Geometry check sheet. Reference: the model listing, model coordinates, mm. Face numbers are marked on the shaded views. Give positions to 0.01 mm unless a question says otherwise; leave off trailing zeros. Write each loop counter-clockwise with the first axis right and the second up, starting at its lowest first coordinate (ties: lowest second). Pieces come first, ordered by that corner, then holes. Notation, with made-up numbers: M -19,33.5 L 0,33.5 A16 cw 0,46.5 Z; hole C 9.5,87.25 d11. An arc over 180 degrees is marked long. Write each question's results on one line, items separated by ' | '.
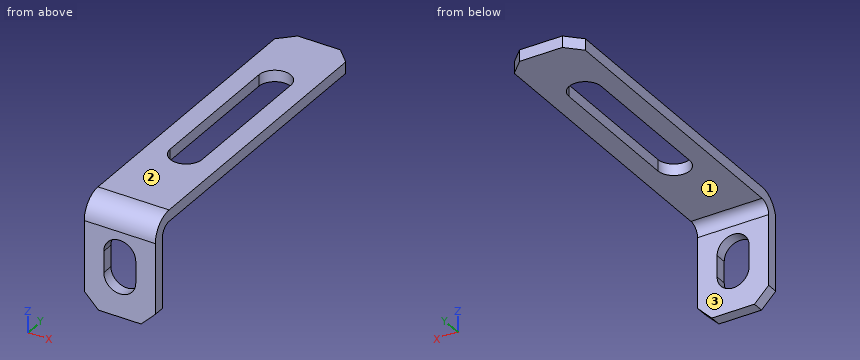
```python
from build123d import *

# Parameters (mm, degrees)
SKETCH1_W           = 15
SKETCH1_H           = 45
BOSS_EXTRUDE1_DEPTH = 10
SKETCH2_W           = 13.4
SKETCH2_H           = 43.4
CUT_EXTRUDE1_DEPTH  = 49.476798574
CUT_EXTRUDE2_DEPTH  = 47.995318916
CUT_EXTRUDE3_DEPTH  = 49.476798574
CHAMFER1_SIZE       = 2
FILLET1_R           = 1.5
FILLET2_R           = 3.1


with BuildPart() as part:
    # Sketch1 → Boss-Extrude1 (new body)
    with BuildSketch(Plane(origin=(10, 0, 0), x_dir=(0, 0, -1), z_dir=(1, 0, 0))):
        with Locations((7.5, 22.5)):
            Rectangle(SKETCH1_W, SKETCH1_H)
    extrude(amount=-BOSS_EXTRUDE1_DEPTH)

    # Sketch2 → Cut-Extrude1 (cut, through all)
    with BuildSketch(Plane.ZY):
        with Locations((-8.3, 23.3)):
            Rectangle(SKETCH2_W, SKETCH2_H)
    extrude(amount=-CUT_EXTRUDE1_DEPTH, mode=Mode.SUBTRACT)

    # Sketch3 → Cut-Extrude2 (cut, through all)
    with BuildSketch(Plane(origin=(0, 1.6, 0), x_dir=(-1, 0, 0), z_dir=(0, 1, 0))):
        with BuildLine():
            Line((-2.75, -9.5), (-2.75, -6.5))
            ThreePointArc((-2.75, -6.5), (-5, -4.25), (-7.25, -6.5))
            Line((-7.25, -6.5), (-7.25, -9.5))
            ThreePointArc((-7.25, -9.5), (-5, -11.75), (-2.75, -9.5))
        make_face()
    extrude(amount=-CUT_EXTRUDE2_DEPTH, mode=Mode.SUBTRACT)

    # Sketch4 → Cut-Extrude3 (cut, through all)
    with BuildSketch(Plane.XY):
        with BuildLine():
            Line((7.25, 15), (7.25, 35))
            ThreePointArc((7.25, 35), (5, 37.25), (2.75, 35))
            Line((2.75, 35), (2.75, 15))
            ThreePointArc((2.75, 15), (5, 12.75), (7.25, 15))
        make_face()
    extrude(amount=-CUT_EXTRUDE3_DEPTH, mode=Mode.SUBTRACT)

    # Chamfer1
    chamfer1_edges = [part.edges().sort_by_distance(p)[0] for p in [
        (0, 0.8, -15),
        (10, 45, -0.8),
        (0, 45, -0.8),
        (10, 0.8, -15),
    ]]
    chamfer(chamfer1_edges, length=CHAMFER1_SIZE)

    # Fillet1
    fillet1_edges = [part.edges().sort_by_distance(p)[0] for p in [
        (5, 1.6, -1.6),
    ]]
    fillet(fillet1_edges, radius=FILLET1_R)

    # Fillet2
    fillet2_edges = [part.edges().sort_by_distance(p)[0] for p in [
        (5, 0, 0),
    ]]
    fillet(fillet2_edges, radius=FILLET2_R)


solid = part.part
```
Q1. Release check for a two-part mould opening along Z. For the marked faces 1, 2 and 3 record: released by +Z, released by -Z, zero draft, split by the parting line, or undercut.
Answer key:
face 1: released by -Z | face 2: released by +Z | face 3: zero draft
Q2. Section check C-C (x = 9.25). Enter the section's corners in (y, z), then the cut area to 3 significant figures.
Answer key:
outline: M 0,-13.75 L 1.6,-13.75 L 1.6,-3.1 A1.5 cw 3.1,-1.6 L 43.75,-1.6 L 43.75,0 L 3.1,0 A3.1 ccw 0,-3.1 Z | area: 87.9 mm2
Q3. Section check A-A (x = 5). Enter the section's corners in (y, z).
Answer key:
outline: M 0,-15 L 1.6,-15 L 1.6,-11.75 L 0,-11.75 Z; M 0,-4.25 L 1.6,-4.25 L 1.6,-3.1 A1.5 cw 3.1,-1.6 L 12.75,-1.6 L 12.75,0 L 3.1,0 A3.1 ccw 0,-3.1 Z; M 37.25,-1.6 L 45,-1.6 L 45,0 L 37.25,0 Z
Q4. Section check D-D (y = 5). Enter the section's corners in (x, z), then the cut area to 3 significant figures.
Answer key:
outline: M 0,-1.6 L 10,-1.6 L 10,0 L 0,0 Z | area: 16.0 mm2
Q5. Material ranges on probe 1 along X at (y, z) = (16.5, -0.75); probe 2 along Y at (x, z) = (9.5, -5.25); probe 3 along Z at (x, y) = (3.5, 13), recorded low to high. Write a range as [from, to].
Answer key:
probe 1: x = [0, 2.75], [7.25, 10] | probe 2: y = [0, 1.6] | probe 3: z = [-1.6, 0]
Q6. Depth check by flat-ended pin: P1, Ø3, axis at x = 2.5, y = 26.5, coming from the +Z side; P2, Ø8, axis at y = 38, z = -7.5, coming from the -X side; P3, Ø5, axis at x = 4, z = -7, coming from the +Y side. Enter the tip coordinate at first touch or a pass-through.
Answer key:
P1: stops at z = 0 | P2: passes through | P3: stops at y = 1.6
Q7. Section check B-B (y = 32.5). Enter the section's corners in (x, z), then the cut area to 3 significant figures.
Answer key:
outline: M 0,-1.6 L 2.75,-1.6 L 2.75,0 L 0,0 Z; M 7.25,-1.6 L 10,-1.6 L 10,0 L 7.25,0 Z | area: 8.80 mm2
